Can you work these out from the model? Positions are in its coordinate system, mm. A direction names the side the tool comes from. Give positions to 0.01 mm unless a question says otherwise; leave off trailing zeros. Write each loop counter-clockwise with the first axis right and the second up, starting at its lowest first coordinate (ties: lowest second). Pieces come first, ordered by that corner, then holes.
from build123d import *

# Parameters (mm, degrees)
F0_R     = 3.175
F1_DEPTH = 38.1
F3_W     = 127
F3_H     = 25.4
F4_DEPTH = 95.251
F6_DEPTH = 38.101
F7_R     = 6.35
F8_R     = 6.34999


# Not quite as in the source:
# - a fillet or chamfer is up to 0.001 mm smaller than in the source, because OpenCascade refuses the exact size


with BuildPart() as f1:
    # F0 (on Front) → F1 (new body)
    with BuildSketch(Plane.XZ):
        with BuildLine():
            Line((-49.5749215348, 67.2876468139), (-105.8131025593, -30.1197400458))
            Line((-105.8131025593, -30.1197400458), (21.1868974407, -30.1197400458))
            Line((21.1868974407, -30.1197400458), (-35.0512835838, 67.2876468139))
            ThreePointArc((-35.0512835838, 67.2876468139), (-42.3131025593, 71.4802599542), (-49.5749215348, 67.2876468139))
        make_face()
        with Locations((-42.3131025593, 63.0950336736)):
            Circle(F0_R, mode=Mode.SUBTRACT)
    extrude(amount=F1_DEPTH)

    # F3 (on offset) → F4 (cut, through all)
    with BuildSketch(Plane(origin=(0, 0, -23.7697400458), x_dir=(1, 0, 0), z_dir=(0, 0, -1))):
        with Locations((-42.3131025593, 19.05)):
            Rectangle(F3_W, F3_H)
    extrude(amount=-F4_DEPTH, mode=Mode.SUBTRACT)

    # F5 (on face) → F6 (cut, through all)
    with BuildSketch(Plane.XZ.offset(38.1)):
        Polygon((-0.8101478154, -17.4197400458), (-42.3131025593, 54.4654862348), (-83.8160573032, -17.4197400458), align=None)
    extrude(amount=-F6_DEPTH, mode=Mode.SUBTRACT)

    # F7
    f7_edges = [f1.edges().sort_by_distance(p)[0] for p in [
        (-42.313103, -34.925, 54.465486),
        (-83.816057, -34.925, -17.41974),
        (-0.810148, -34.925, -17.41974),
        (-0.810148, -3.175, -17.41974),
        (-83.816057, -3.175, -17.41974),
        (-42.313103, -3.175, 54.465486),
    ]]
    fillet(f7_edges, radius=F7_R)

    # F8 (radius 6.35 in the source; OpenCascade refuses exactly that, so slightly less here)
    f8_edges = [f1.edges().sort_by_distance(p)[0] for p in [
        (-42.313103, -6.35, -23.76974),
        (-42.313103, -31.75, -23.76974),
    ]]
    fillet(f8_edges, radius=F8_R)


solid = f1.part
(1) Imagine slicing it at B-B, the plane z = 54.5. Write out the boundary of the cut face in (x, y), plus the area to 3 significant figures.
Returned:
outline: (-56.96, -38.1) - (-27.67, -38.1) - (-27.67, -31.75) - (-56.96, -31.75) - close; (-56.96, -6.35) - (-27.67, -6.35) - (-27.67, 0) - (-56.96, 0) - close
area: 372 mm2
(2) Imagine slicing it at C-C, the plane y = -23. Write out the boundary of the cut face in (x, z).
Returned:
outline: (-105.81, -30.12) - (21.19, -30.12) - (17.52, -23.77) - (-102.15, -23.77) - close
(3) If we mould it in two halves opening along Z, with no side actions, what happens to faces 1 (the face through (-42.22, -3.131, 48.115)), 2 (the face through (-83.55, -6.08, 8.44)), 3 (the face through (-43, 0, -20))? For each: +Z half, -Z half, draft (parallel to the pull), parting line (faces both ways), or undercut.
Returned:
face 1: undercut
face 2: +Z half
face 3: draft
(4) If I drill on L1, parallel to Y at x = -85, z = -12.5; L2, parallel to Z at x = -69, y = -16.5; L3, parallel to X at y = -4, z = 28, over which ranges is the centre line in solid material (lowest first)?
Returned:
L1: y = -38.1 to -31.75, -6.35 to 0
L2: z = -30.12 to -23.77
L3: x = -72.26 to -57.59, -27.03 to -12.37
(5) Imagine slicing it at A-A, the plane x = -65.5. Give the number of separate pieces and of enclosed holes in the cut face, plus the area to 3 significant figures.
Returned:
separate pieces: 3
enclosed holes: 0
area: 662 mm2
(6) Imagine slicing it at D-D, the plane z = 41. Write out the boundary of the cut face in (x, y), plus the area to 3 significant figures.
Returned:
outline: (-64.75, -38.1) - (-50.09, -38.1) - (-50.09, -31.75) - (-64.75, -31.75) - close; (-64.75, -6.35) - (-50.09, -6.35) - (-50.09, 0) - (-64.75, 0) - close; (-34.54, -38.1) - (-19.87, -38.1) - (-19.87, -31.75) - (-34.54, -31.75) - close; (-34.54, -6.35) - (-19.87, -6.35) - (-19.87, 0) - (-34.54, 0) - close
area: 372 mm2
(7) Will these pins go through, and if not, where does the flat tip stop? P1, Ø5, axis at x = -29.5, y = -3, coming from the +Z side; P2, Ø4, axis at x = -55, y = -21, coming from the +Z side; P3, Ø3, axis at x = -31, y = -35.5, coming from the +Z side.
Returned:
P1: stops at z = 62
P2: stops at z = -23.77
P3: stops at z = 62.87
(8) For faces 4 (the face through (-41.5, -8.2, -21.9)), 5 (the face through (-0.3, -6.1, 7.1)), 6 (the face through (-21.348, -3.219, 18.153)), which set-ups out of +Z, -Z, +X, -X, +Y, -Y let a thin tool reach every point of the face, with its end or its side?
Returned:
face 4: +Z, +X, -X
face 5: +Z, +X, +Y, -Y
face 6: +Y, -Y
